Can you work these out from the model? Positions are in its coordinate system, mm. A direction names the side the tool comes from. Coordinates: 2 decimals unless noted, no trailing zeros. Order: outer loops, then holes, each group sorted by start corner. A loop starts at its lowest first (then second) coordinate and runs counter-clockwise, first axis right, second up. Notation, with made-up numbers: (-36, -8.75) -> (8, -8.75) arc R24 cw to (8, 3.25) -> close; hole circle Ø8 at (24.25, 67.25). An arc over 180 degrees is marked (long way). Use a Markdown table: item, result. Add a question column.
1. Suppose I cut it at D-D, the plane x = -106.5. List the corners of the cut face in (y, z) for me, then the cut area to 3 significant figures.
2. For faces 1 (the flat face through (137, 75, 0)), 2 (the flat face through (-4, -317.5, 16)), which set-ups out of +Z, -Z, +X, -X, +Y, -Y let a thin tool reach every point of the face, with its end or its side?
3. Suppose I cut it at C-C, the plane y = 0. List the corners of the cut face in (x, z) for me (3 decimals).
4. If I drill on line 1 along X through (y, z) = (279, 16); line 2 along Y through (x, z) = (0, -254) (3 decimals), over which ranges is the centre line in solid material (lowest first)? Write a range as from..to.
5. For pin 1 Ø12 at (y, z) = (102, -449.5) entering from -X; pin 2 Ø5 at (y, z) = (-19.5, -345.5) entering from -X; pin 3 Ø3 at (y, z) = (-88.5, -181.5) entering from +X, each with a flat end and sliding along its axis, tell me the tip position at first contact or that it passes through.
6. We'd pull the mould along X, two halves only. Please class faces 3 (the cylindrical face through (-310.26, -309.86, 15.65)), 4 (the cylindrical face through (310.26, 309.86, 15.65)), 5 (the cylindrical face through (-268.8, -276.06, 15.65)): pulls with the +X half, pulls with the -X half, needs draft (parallel to the pull), parting line crosses it, or undercut.
7. Suppose I cut it at A-A, the plane x = 279.4. List the corners of the cut face in (y, z) for me.
```python
from build123d import *

# Parameters (mm, degrees)
F0_R     = 11.1125
F1_DEPTH = 31.75
F2_R     = 149.225
F2_R_2   = 136.525
F3_DEPTH = 609.6
F4_R     = 136.525
F5_DEPTH = 50.8


with BuildPart() as f1:
    # F0 (on Top) → F1 (new body)
    with BuildSketch(Plane.XY):
        with BuildLine():
            ThreePointArc((317.5, 292.1), (310.060512, 310.060512), (292.1, 317.5))
            Line((292.1, 317.5), (-292.1, 317.5))
            ThreePointArc((-292.1, 317.5), (-310.060512, 310.060512), (-317.5, 292.1))
            Line((-317.5, 292.1), (-317.5, -292.1))
            ThreePointArc((-317.5, -292.1), (-310.060512, -310.060512), (-292.1, -317.5))
            Line((-292.1, -317.5), (292.1, -317.5))
            ThreePointArc((292.1, -317.5), (310.060512, -310.060512), (317.5, -292.1))
            Line((317.5, -292.1), (317.5, 292.1))
        make_face()
        with Locations((-279.4, -279.4)):
            Circle(F0_R, mode=Mode.SUBTRACT)
        with Locations((279.4, -279.4)):
            Circle(F0_R, mode=Mode.SUBTRACT)
        with Locations((-279.4, 279.4)):
            Circle(F0_R, mode=Mode.SUBTRACT)
        with Locations((279.4, 279.4)):
            Circle(F0_R, mode=Mode.SUBTRACT)
    extrude(amount=F1_DEPTH)

    # F2 (on face) → F3 (join)
    with BuildSketch(Plane(origin=(0, 0, 0), x_dir=(1, 0, 0), z_dir=(0, 0, -1))):
        Circle(F2_R)
        Circle(F2_R_2, mode=Mode.SUBTRACT)
    extrude(amount=F3_DEPTH)

    # F4 (on face) → F5 (cut)
    with BuildSketch(Plane.XY.offset(31.75)):
        Circle(F4_R)
    extrude(amount=-F5_DEPTH, mode=Mode.SUBTRACT)


solid = f1.part
```
Worked out:
| question | item | result |
|---|---|---|
| 1 | outline | (-317.5, 0) -> (-104.53, 0) -> (-104.53, -609.6) -> (-85.42, -609.6) -> (-85.42, 31.75) -> (-317.5, 31.75) -> close; (85.42, -609.6) -> (104.53, -609.6) -> (104.53, 0) -> (317.5, 0) -> (317.5, 31.75) -> (85.42, 31.75) -> close |
| 1 | area | 38,000 mm² |
| 2 | face 1 | -Z |
| 2 | face 2 | +Z, -Z, +X, -X, -Y |
| 3 | outline | (-317.5, 0) -> (-149.225, 0) -> (-149.225, -609.6) -> (-136.525, -609.6) -> (-136.525, 31.75) -> (-317.5, 31.75) -> close; (136.525, -609.6) -> (149.225, -609.6) -> (149.225, 0) -> (317.5, 0) -> (317.5, 31.75) -> (136.525, 31.75) -> close |
| 4 | line 1 | x = -317.5..-290.51, -268.29..268.29, 290.51..317.5 |
| 4 | line 2 | y = -149.225..-136.525, 136.525..149.225 |
| 5 | pin 1 | stops at x = -114.25 |
| 5 | pin 2 | stops at x = -148.25 |
| 5 | pin 3 | stops at x = 121.24 |
| 6 | face 3 | pulls with the -X half |
| 6 | face 4 | pulls with the +X half |
| 6 | face 5 | undercut |
| 7 | outline | (-317.5, 0) -> (-290.51, 0) -> (-290.51, 31.75) -> (-317.5, 31.75) -> close; (-268.29, 0) -> (268.29, 0) -> (268.29, 31.75) -> (-268.29, 31.75) -> close; (290.51, 0) -> (317.5, 0) -> (317.5, 31.75) -> (290.51, 31.75) -> close |
